Could you check a few things on this model? Use its own coordinates, in mm. Coordinates: 2 decimals unless noted, no trailing zeros. Order: outer loops, then holes, each group sorted by start corner. A loop starts at its lowest first (then second) coordinate and runs counter-clockwise, first axis right, second up.
```python
from build123d import *

# Parameters (mm, degrees)
SKETCH1_W               = 152.4
SKETCH1_H               = 152.4
BOSS_EXTRUDE1_DEPTH     = 6.35
SKETCH2_R               = 4.1656
SKETCH2_R_2             = 3.175
CUT_EXTRUDE1_DEPTH      = 1
CUT_EXTRUDE1_DEPTH_BACK = 7.35


with BuildPart() as part:
    # Sketch1 → Boss-Extrude1 (new body)
    with BuildSketch(Plane(origin=(0, 0, 0), x_dir=(1, 0, 0), z_dir=(0, 1, 0))):
        with Locations((76.2, 76.2)):
            Rectangle(SKETCH1_W, SKETCH1_H)
    extrude(amount=BOSS_EXTRUDE1_DEPTH)

    # Sketch2 → Cut-Extrude1 (cut, two sides)
    with BuildSketch(Plane(origin=(0, 6.35, 0), x_dir=(1, 0, 0), z_dir=(0, 1, 0))) as cut_extrude1_sk:
        with Locations((19.05, 38.1)):
            Circle(SKETCH2_R)
        with Locations((19.05, 114.3)):
            Circle(SKETCH2_R)
        with Locations((133.35, 114.3)):
            Circle(SKETCH2_R)
        with Locations((133.35, 38.1)):
            Circle(SKETCH2_R)
        with Locations((104.484271247, 104.484271247)):
            Circle(SKETCH2_R_2)
        with Locations((47.915728753, 47.915728753)):
            Circle(SKETCH2_R_2)
        with Locations((47.915728753, 104.484271247)):
            Circle(SKETCH2_R_2)
        with Locations((104.484271247, 47.915728753)):
            Circle(SKETCH2_R_2)
    extrude(amount=CUT_EXTRUDE1_DEPTH, mode=Mode.SUBTRACT)
    extrude(cut_extrude1_sk.sketch, amount=-CUT_EXTRUDE1_DEPTH_BACK, mode=Mode.SUBTRACT)


solid = part.part
```
Item 1: Suppose I cut it at B-B (x = 133.35). List the corners of the cut face in (y, z) for me.
Item 2: Suppose I cut it at A-A (z = -114.3). List the corners of the cut face in (x, y) for me.
Item 3: Thinking about a two-plate mould opening in X: for faces 1 (the face through (75, 3, -152.4)), 2 (the face through (152.4, 3, -75)), 3 (the face through (18.51, 3.22, -118.43)), 4 (the face through (0, 3, -75)), which applies, +X half, -X half, draft (parallel to the pull), parting line (faces both ways), or undercut?
Item 4: I need wall thicknesses on line 1 (X direction, y = 1.75, z = -114.3); line 2 (Z direction, x = 133.35, y = 2.75); line 3 (Z direction, x = 49, y = 2.5). Which ranges of each line are inside material? Lowest first, please.
Geometry results:
1. outline: (0, -152.4) - (6.35, -152.4) - (6.35, -118.47) - (0, -118.47) - close; (0, -110.13) - (6.35, -110.13) - (6.35, -42.27) - (0, -42.27) - close; (0, -33.93) - (6.35, -33.93) - (6.35, 0) - (0, 0) - close
2. outline: (0, 0) - (14.88, 0) - (14.88, 6.35) - (0, 6.35) - close; (23.22, 0) - (129.18, 0) - (129.18, 6.35) - (23.22, 6.35) - close; (137.52, 0) - (152.4, 0) - (152.4, 6.35) - (137.52, 6.35) - close
3. face 1: draft
3. face 2: +X half
3. face 3: undercut
3. face 4: -X half
4. line 1: x = 0 to 14.88, 23.22 to 129.18, 137.52 to 152.4
4. line 2: z = -152.4 to -118.47, -110.13 to -42.27, -33.93 to 0
4. line 3: z = -152.4 to -107.47, -101.5 to -50.9, -44.93 to 0
